Here's how the part is built. I have some questions about the finished solid (model axes, mm). A direction names the side the tool comes from. Coordinates: 2 decimals unless noted, no trailing zeros. Write each loop counter-clockwise with the first axis right and the second up, starting at its lowest first coordinate (ties: lowest second). Pieces come first, ordered by that corner, then holes. Notation, with made-up numbers: (25.5, 49.5) -> (62.5, 49.5) arc R24 cw to (62.5, 61.5) -> close; hole circle Ø1 at (-27.75, 36.5). An arc over 180 degrees is marked (long way). Put each result on its own line as item: value. Start each with the question number.
Item 1: If we mould it in two halves opening along Y, with no side actions, what happens to faces 4 (the face through (-7.6, -64.8, 7.4)), 5 (the face through (35, 6.213, 9)), 6 (the face through (7.6, 64.8, 7.4))? For each: released by +Y, released by -Y, zero draft, split by the parting line, or undercut.
Item 2: I want a section at D-D, the plane y = -19.5. List the corners of the cut face in (x, z) for me.
Item 3: I want a section at B-B, the plane x = 55.5. List the corners of the cut face in (y, z) for me.
Item 4: I need wall thicknesses on line 1 (Y direction, x = 12.5, z = 10); line 2 (Y direction, x = -14, z = 11.25); line 3 (X direction, y = 42, z = 8.5). Which ranges of each line are inside material? Lowest first, please. Write a range as [from, to].
Item 5: For pin 1 (1.5 mm diameter, centred on x = -13, z = 7.5, fed in from +Y); pin 2 (1.6 mm diameter, centred on y = -7, z = 11.5, fed in from -X); pin 3 (12 mm diameter, centred on x = -27.5, y = 34.5, fed in from +Z); pin 4 (4 mm diameter, centred on y = -10.5, z = 8, fed in from -X), each with a flat end and sliding along its axis, tell me the tip position at first contact or that it passes through.
Item 6: I want a section at C-C, the plane x = 19. List the corners of the cut face in (y, z) for me.
Item 7: I want a section at A-A, the plane y = -37.5. List the corners of the cut face in (x, z) for me.
Item 8: On a 3-axis mill with a long thin cutter (end or side, diameter ignored), from which of +Z, -Z, +X, -X, +Y, -Y can I reach the whole of each face in a straight line? I mean faces 1 (the face through (41.66, -48.17, 8.92)), 2 (the face through (7.4, -65.2, 7.4)), 3 (the face through (33.73, -18.8, 7.4)). Say none if no direction works.
from build123d import *

# Parameters (mm, degrees)
F1_DEPTH = 10
F2_DEPTH = 5
F3_T     = -3


with BuildPart() as f1:
    # F0 (on Top) → F1 (new body)
    with BuildSketch(Plane.XY):
        Polygon((-24.1421356237, 9.2129365882), (-50, 9.2129365882), (-50, 14.2129365882), (-80, 0), (-50, 0), (0, 0), (0, 50), (0, 80), (-15, 50), (-10, 50), (-10, 23.3550722119), (-10, 9.2129365882), align=None)
        Polygon((-43.0507218531, 28.1215228176), (-24.1421356237, 9.2129365882), (-10, 9.2129365882), (-35.9796540413, 35.1925906294), align=None)
        Polygon((-35.9796540413, 35.1925906294), (-10, 9.2129365882), (-10, 23.3550722119), (-28.9085862294, 42.2636584413), align=None)
        Polygon((-46.5862557591, 24.5859889116), (-43.0507218531, 28.1215228176), (-35.9796540413, 35.1925906294), (-57.5228781318, 56.73581472), align=None)
        Polygon((-50, 0), (-80, 0), (-50, -14.2129365882), (-50, -9.2129365882), (-24.1421356237, -9.2129365882), (-10, -9.2129365882), (-10, -23.3550722119), (-10, -50), (-15, -50), (0, -80), (0, -50), (0, 0), align=None)
        Polygon((-57.5228781318, 56.73581472), (-35.9796540413, 35.1925906294), (-28.9085862294, 42.2636584413), (-25.3730523235, 45.7991923472), align=None)
        Polygon((0, 50), (0, 0), (50, 0), (80, 0), (50, 14.2129365882), (50, 9.2129365882), (24.1421356237, 9.2129365882), (10, 9.2129365882), (10, 23.3550722119), (10, 50), (15, 50), (0, 80), align=None)
        Polygon((50, 0), (0, 0), (0, -50), (0, -80), (15, -50), (10, -50), (10, -23.3550722119), (10, -9.2129365882), (24.1421356237, -9.2129365882), (50, -9.2129365882), (50, -14.2129365882), (80, 0), align=None)
        Polygon((-10, -9.2129365882), (-24.1421356237, -9.2129365882), (-43.0507218531, -28.1215228176), (-35.9796540413, -35.1925906294), align=None)
        Polygon((-10, -23.3550722119), (-10, -9.2129365882), (-35.9796540413, -35.1925906294), (-28.9085862294, -42.2636584413), align=None)
        Polygon((-35.9796540413, -35.1925906294), (-43.0507218531, -28.1215228176), (-46.5862557591, -24.5859889116), (-57.5228781318, -56.73581472), align=None)
        Polygon((-28.9085862294, -42.2636584413), (-35.9796540413, -35.1925906294), (-57.5228781318, -56.73581472), (-25.3730523235, -45.7991923472), align=None)
        Polygon((28.9085862294, 42.2636584413), (10, 23.3550722119), (10, 9.2129365882), (35.9796540413, 35.1925906294), align=None)
        Polygon((10, 9.2129365882), (24.1421356237, 9.2129365882), (43.0507218531, 28.1215228176), (35.9796540413, 35.1925906294), align=None)
        Polygon((43.0507218531, -28.1215228176), (24.1421356237, -9.2129365882), (10, -9.2129365882), (35.9796540413, -35.1925906294), align=None)
        Polygon((10, -9.2129365882), (10, -23.3550722119), (28.9085862294, -42.2636584413), (35.9796540413, -35.1925906294), align=None)
        Polygon((25.3730523235, 45.7991923472), (28.9085862294, 42.2636584413), (35.9796540413, 35.1925906294), (57.5228781318, 56.73581472), align=None)
        Polygon((35.9796540413, 35.1925906294), (43.0507218531, 28.1215228176), (46.5862557591, 24.5859889116), (57.5228781318, 56.73581472), align=None)
        Polygon((46.5862557591, -24.5859889116), (43.0507218531, -28.1215228176), (35.9796540413, -35.1925906294), (57.5228781318, -56.73581472), align=None)
        Polygon((35.9796540413, -35.1925906294), (28.9085862294, -42.2636584413), (25.3730523235, -45.7991923472), (57.5228781318, -56.73581472), align=None)
    extrude(amount=F1_DEPTH)

    # F2 (add): a face of the model
    f2_faces = [f1.faces().sort_by_distance(p)[0] for p in [
        (0, 0, 10),
    ]]
    extrude(f2_faces, amount=F2_DEPTH)

    # F3
    f3_openings = [f1.faces().sort_by_distance(p)[0] for p in [
        (0, 0, 15),
    ]]
    offset(amount=F3_T, openings=f3_openings, kind=Kind.INTERSECTION)


solid = f1.part
Calculated:
1. face 4: released by -Y
1. face 5: undercut
1. face 6: released by +Y
2. outline: (-34.43, 0) -> (34.43, 0) -> (34.43, 15) -> (30.19, 15) -> (30.19, 3) -> (10.39, 3) -> (10.39, 15) -> (7, 15) -> (7, 3) -> (-7, 3) -> (-7, 15) -> (-10.39, 15) -> (-10.39, 3) -> (-30.19, 3) -> (-30.19, 15) -> (-34.43, 15) -> close
3. outline: (-56.05, 0) -> (-50.79, 0) -> (-50.79, 15) -> (-56.05, 15) -> close; (-11.61, 0) -> (11.61, 0) -> (11.61, 15) -> (8.29, 15) -> (8.29, 3) -> (-8.29, 3) -> (-8.29, 15) -> (-11.61, 15) -> close; (50.79, 0) -> (56.05, 0) -> (56.05, 15) -> (50.79, 15) -> close
4. line 1: y = [-55, -50], [-25.86, -21.61], [21.61, 25.86], [50, 55]
4. line 2: y = [-52, -50], [-27.36, -23.11], [23.11, 27.36], [50, 52]
4. line 3: x = [-52.51, -49.34], [-32.89, -28.64], [-10, -7], [7, 10], [28.64, 32.89], [49.34, 52.51]
5. pin 1: stops at y = 55.5
5. pin 2: stops at x = -66.91
5. pin 3: stops at z = 15
5. pin 4: stops at x = -62.06
6. outline: (-32.36, 0) -> (32.36, 0) -> (32.36, 15) -> (28.11, 15) -> (28.11, 3) -> (8.31, 3) -> (8.31, 15) -> (6.21, 15) -> (6.21, 3) -> (-6.21, 3) -> (-6.21, 15) -> (-8.31, 15) -> (-8.31, 3) -> (-28.11, 3) -> (-28.11, 15) -> (-32.36, 15) -> close
7. outline: (-50.98, 0) -> (-24.14, 0) -> (-24.14, 15) -> (-28.39, 15) -> (-28.39, 3) -> (-47.81, 3) -> (-47.81, 15) -> (-50.98, 15) -> close; (-10, 0) -> (10, 0) -> (10, 15) -> (7, 15) -> (7, 3) -> (-7, 3) -> (-7, 15) -> (-10, 15) -> close; (24.14, 0) -> (50.98, 0) -> (50.98, 15) -> (47.81, 15) -> (47.81, 3) -> (28.39, 3) -> (28.39, 15) -> (24.14, 15) -> close
8. face 1: +Z
8. face 2: +Z, -Z, -Y
8. face 3: +Z, -Z
